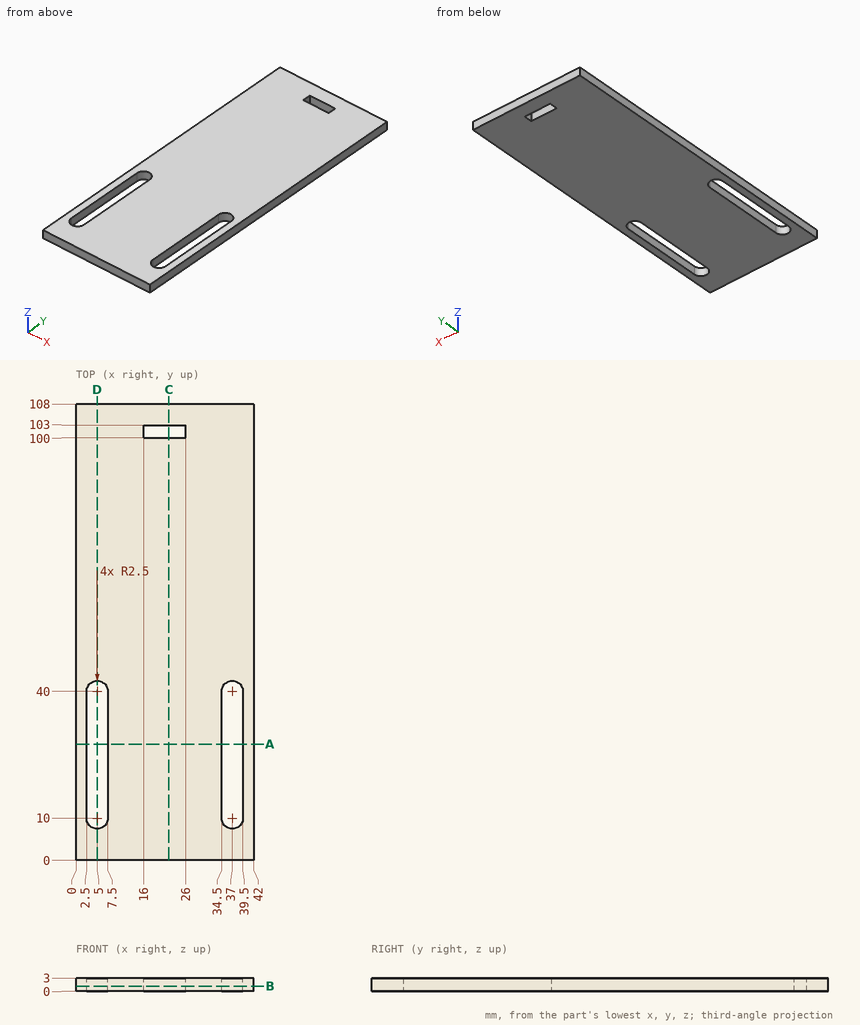
Job drawing, mm, ordinate dimensions from the low corner. One solid piece. Round coordinates to 2 decimals unless told otherwise and drop trailing zeros. Order: outer loops, then holes, each group sorted by start corner. A loop starts at its lowest first (then second) coordinate and runs counter-clockwise, first axis right, second up. Notation, with made-up numbers: M 19.5,-34.5 L 49.5,-34.5 A25 cw 49.5,-21.5 Z; hole C 59,14.5 d11. An arc over 180 degrees is marked long. Write each question's results on one line, items separated by ' | '. Start each with the question number.
(1) Saw through at C-C, the plane x = 22. Give the cut face in (y, z).
(2) Probe probe 1 along X at (y, z) = (20.5, 2.85); probe 2 along Y at (x, z) = (24.5, 1.6); probe 3 along X at (y, z) = (100.5, 0.5). List the from-to ranges inside material, lowest first. Write a range as from..to.
(3) Saw through at A-A, the plane y = 27.5. Give the cut face in (x, z).
(4) Saw through at B-B, the plane z = 1.2. Give the cut face in (x, y), then the cut area to 3 significant figures.
(5) Saw through at D-D, the plane x = 5. Give the cut face in (y, z).
Established:
1) outline: M 0,0 L 100,0 L 100,3 L 0,3 Z; M 103,0 L 108,0 L 108,3 L 103,3 Z
2) probe 1: x = 0..2.5, 7.5..34.5, 39.5..42 | probe 2: y = 0..100, 103..108 | probe 3: x = 0..16, 26..42
3) outline: M 0,0 L 2.5,0 L 2.5,3 L 0,3 Z; M 7.5,0 L 34.5,0 L 34.5,3 L 7.5,3 Z; M 39.5,0 L 42,0 L 42,3 L 39.5,3 Z
4) outline: M 0,0 L 42,0 L 42,108 L 0,108 Z; hole M 2.5,10 A2.5 ccw 7.5,10 L 7.5,40 A2.5 ccw 2.5,40 Z; hole M 16,100 L 26,100 L 26,103 L 16,103 Z; hole M 34.5,10 A2.5 ccw 39.5,10 L 39.5,40 A2.5 ccw 34.5,40 Z | area: 4,170 mm^2
5) outline: M 0,0 L 7.5,0 L 7.5,3 L 0,3 Z; M 42.5,0 L 108,0 L 108,3 L 42.5,3 Z
